Could you check a few things on this drawing? It's one solid part, dimensions in mm from its lowest x, y, z. A direction names the side the tool comes from. Coordinates: 2 decimals unless noted, no trailing zeros. Write each loop counter-clockwise with the first axis right and the second up, starting at its lowest first coordinate (ties: lowest second). Pieces come first, ordered by that corner, then holes.
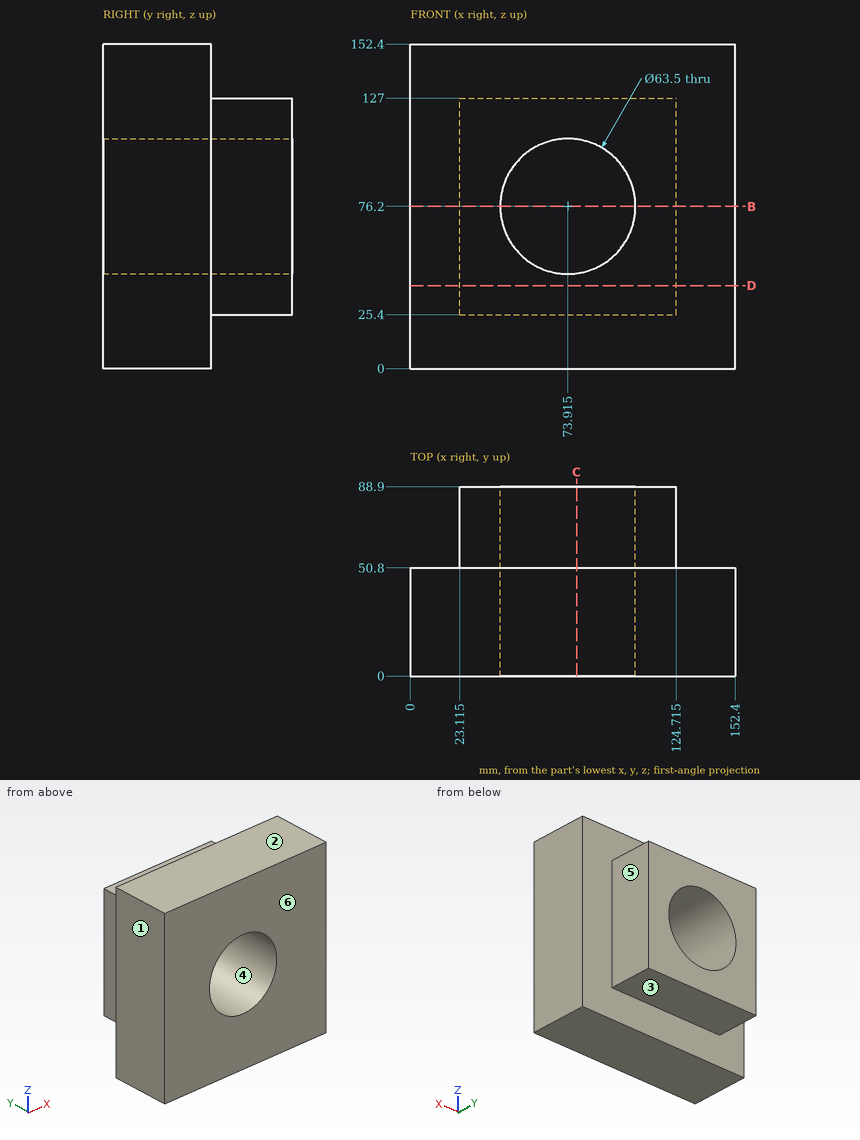
1) Imagine slicing it at C-C on x = 78. Please give me the cut outline in (y, z).
Values follow:
outline: (0, 0) - (50.8, 0) - (50.8, 25.4) - (88.9, 25.4) - (88.9, 44.71) - (0, 44.71) - close; (0, 107.69) - (88.9, 107.69) - (88.9, 127) - (50.8, 127) - (50.8, 152.4) - (0, 152.4) - close
2) We'd pull the mould along Z, two halves only. Please class the marked faces 1, 2, 3 and 4: pulls with the +Z half, pulls with the -Z half, needs draft (parallel to the pull), parting line crosses it, or undercut.
Values follow:
face 1: needs draft
face 2: pulls with the +Z half
face 3: pulls with the -Z half
face 4: undercut
3) Imagine slicing it at D-D on z = 39. Please give me the cut outline in (x, y) (1 decimal).
Values follow:
outline: (0, 0) - (152.4, 0) - (152.4, 50.8) - (124.7, 50.8) - (124.7, 88.9) - (23.1, 88.9) - (23.1, 50.8) - (0, 50.8) - close
4) On a 3-axis mill with a long thin cutter (end or side, diameter ignored), from which of +Z, -Z, +X, -X, +Y, -Y can I reach the whole of each face in a straight line? I mean the marked faces 5 and 6. Say none if no direction works.
Values follow:
face 5: +Z, -Z, +X, +Y
face 6: +Z, -Z, +X, -X, -Y
5) Imagine slicing it at B-B on z = 76.2. Please give me the cut outline in (x, y) (1 decimal).
Values follow:
outline: (0, 0) - (42.2, 0) - (42.2, 88.9) - (23.1, 88.9) - (23.1, 50.8) - (0, 50.8) - close; (105.7, 0) - (152.4, 0) - (152.4, 50.8) - (124.7, 50.8) - (124.7, 88.9) - (105.7, 88.9) - close
6) Will these pins go through, and if not, where does the flat tip stop? pin 1 (12 mm diameter, centred on y = 71.5, z = 41.5, fed in from -X) (1 decimal); pin 2 (19 mm diameter, centred on x = 82, y = 75, fed in from -Z); pin 3 (1 mm diameter, centred on x = 122.5, y = 71.5, fed in from +Z).
Values follow:
pin 1: stops at x = 23.1
pin 2: stops at z = 25.4
pin 3: stops at z = 127
7) I need wall thicknesses on probe 1 along Z at (x, y) = (39, 67.5); probe 2 along X at (y, z) = (54, 76) (1 decimal); probe 3 along Y at (x, z) = (93.5, 24.5). Which ranges of each line are inside material? Lowest first, please.
Values follow:
probe 1: z = 25.4 to 127
probe 2: x = 23.1 to 42.2, 105.7 to 124.7
probe 3: y = 0 to 50.8
